Check sheet for the modelled part. Datum: model origin and axes. Units: mm. A direction names the side the tool comes from. Coordinates: 2 decimals unless noted, no trailing zeros. Write each loop counter-clockwise with the first axis right and the second up, starting at its lowest first coordinate (ties: lowest second). Pieces come first, ordered by that corner, then holes. Notation, with made-up numbers: M -3.5,26.25 L 0.5,26.25 A10 ccw 0.5,32.25 Z; hole C 27,-17 d2. An arc over 180 degrees is marked long. Answer as CSV lines item,"result". Start each with the question number.
Q1. Thickness scan on line 1 along Z through (x, y) = (-22, 0.45); line 2 along X through (y, z) = (2.5, -37.5); line 3 along X through (y, z) = (0.3, -44.5). Record the ranges inside material, lowest first. Write a range as from..to.
Q2. Depth check by flat-ended pin: pin 1 Ø1 at (x, z) = (-9, -41.5) entering from +Y. Enter the tip coordinate at first touch or a pass-through.
Q3. Access from +Z, -Z, +X, -X, +Y, -Y to the whole of each face (thin tool, end or side, straight path). Record for faces 4 (the cylindrical face through (-15.01, 0.49, -33.54)), 5 (the flat face through (-43, 11, -31)).
Q4. Mould release check, pull along X, two halves, no side actions. Record for faces 1 (the flat face through (-17.6, 1, -31.9)), 2 (the flat face through (0, 11, -32)), 3 (the flat face through (-22, 11, -63)): pulls with the +X half, pulls with the -X half, needs draft (parallel to the pull), parting line crosses it, or undercut.
Q5. Sectioned sample at D-D, the plane z = -58.5. Record the cut outline in (x, y), then the cut area to 3 significant figures.
Q6. Sectioned sample at A-A, the plane z = -44.5. Record the cut outline in (x, y), then the cut area to 3 significant figures.
Q7. Sectioned sample at B-B, the plane x = -22. Record the cut outline in (y, z), then the cut area to 3 significant figures.
Q8. Sectioned sample at C-C, the plane y = 9.25. Record the cut outline in (x, z), then the cut area to 3 significant figures.
Autodesk Fusion 360 part; units mm, degrees
sketch "Sketch1" plane through (0, 0, 0) normal (0, 1, 0) x (1, 0, 0)
  line L0 (0, 0) -> (-44, 0)
  line L1 (-44, 0) -> (-44, 63)
  line L2 (-44, 63) -> (0, 63)
  line L3 (0, 63) -> (0, 0)
  line L4 (-22, 0) -> (-22, 15)
  line L5 (-44, 0) -> (-22, 0)
  line L6 (-22, 0) -> (-22, 63)
  line L7 (-22, 63) -> (-22, 44.5)
  circle A0 centre (-22, 44.5) radius 13
  line L8 (-44, 63) -> (-22, 63)
  line L9 (-5.2012, 3.5077) -> (-38.7988, 3.5077)
  line L10 (-38.7988, 3.5077) -> (-38.7988, 26.4923)
  line L11 (-38.7988, 26.4923) -> (-5.2012, 26.4923)
  line L12 (-5.2012, 26.4923) -> (-5.2012, 3.5077)
  line L13 (-5.2012, 3.5077) -> (-38.7988, 26.4923) construction
  line L14 (-38.7988, 3.5077) -> (-5.2012, 26.4923) construction
  line L15 (-43, 62) -> (-1, 62)
  line L16 (-1, 62) -> (-1, 1)
  line L17 (-1, 1) -> (-43, 1)
  line L18 (-43, 1) -> (-43, 62)
  dimension "d1" = 44
  dimension "d2" = 63
  dimension "d5" = 15
  dimension "d7" = 18.5
  dimension "d8" = 26
  dimension "d9" = 21
  dimension "d13" = 21.5
  dimension "d14" = 1
extrude "Extrude3" add sketch "Sketch1" along normal blind 22 contours L0 L2 L3 L4 L6 L7 L15 L16 L17 | L0 L1 L2 L4 L5 L6 L7 L8 L15 L17 L18 makes body 1
extrude "Extrude2" add sketch "Sketch1" along normal blind 1 separate body contours L0 L2 L3 L4 L6 L7 L15 L16 L17 | L0 L1 L2 L4 L5 L6 L7 L8 L15 L17 L18 | L4 L6 L7 A0 L9 L10 L11 L15 L17 L18 | L4 L6 L7 A0 L9 L11 L12 L15 L16 L17 makes body 2
combine "Combine1" operation add target body 1 tool bodies 2
extrude "Extrude5" add sketch "Sketch1" along normal blind 21 separate body contours L4 L6 L7 A0 L9 L10 L11 L15 L17 L18 | L4 L6 L7 A0 L9 L11 L12 L15 L16 L17 | L4 L6 L9 L10 L11 | L4 L6 L9 L11 L12 | L6 L7 A0 | L6 L7 A0 makes body 3
move_body "Move1" bodies 3 to x (1, 0, 0) y (0, 1, 0) z (0, 0, 1) at (0, 1, 0)
extrude "Extrude6" add sketch "Sketch1" along normal blind -8 and the other way blind -1 separate body contours L6 L7 A0 | L6 L7 A0 makes body 4
combine "Combine2" operation add target body 4 tool bodies 3
sketch "Sketch3" plane through (0, 0, 0) normal (1, 0, 0) x (0, 0, -1)
  line L0 (44.5, -8) -> (44.5, -95.3333)
  line L1 (44.5, -8) -> (44.5007, 25.9882)
  line L2 (44.5, -8) -> (44.5, -13)
  line L3 (44.5, -8) -> (44.5, -13)
  line L4 (44.5, -8) -> (44.5, -13)
  line L5 (44.5, -5.7455) -> (28.5885, -9.273)
  line L6 (44.5, -5.7455) -> (93.193, -5.7455) construction
  line L7 (44.5, -5.7455) -> (101.0974, -5.7455) construction
  line L8 (44.5, -9.273) -> (25, -9.273)
  line L9 (28.5885, -9.273) -> (28.5885, -28.9115)
  line L10 (28.5885, -28.9115) -> (23.5129, -33.9871)
  line L11 (44.5, -13) -> (73.6492, -13) construction
  line L12 (44.5, -13) -> (28.5885, -28.9115)
  line L13 (28.5885, -28.9115) -> (-8.934, -28.9115)
  line L14 (44.5, -13) -> (28.5885, -13)
  line L15 (44.5, -13) -> (7, -12.9775)
  line L16 (7, -12.9775) -> (30.0264, -12.9775) construction
  line L17 (7, -12.9775) -> (-8.934, -28.9115)
  line L18 (-8.934, -28.9115) -> (-8.934, -33.9115)
  line L19 (6.9775, -13) -> (6.9775, -33.9115)
  line L20 (28.5885, -13) -> (6.9775, -13)
  line L21 (-8.934, -28.9115) -> (-8.934, -33.9115)
  line L22 (-8.934, -33.9115) -> (6.9775, -33.9115)
  line L23 (6.9775, -33.9115) -> (44.5, -42.23)
  line L24 (6.9775, -33.9115) -> (31.1364, -33.9115) construction
  line L25 (-8.934, -33.9115) -> (-89.4653, -51.7648)
  line L26 (-8.934, -33.9115) -> (73.5526, -33.9115) construction
  dimension "d31" = 5
  dimension "d36" = 45
  dimension "d37" = 77.5
  dimension "d38" = 37.5
  dimension "d40" = 12.5
  dimension "d41" = 167.5
sketch "Sketch4" plane through (0, 0, 0) normal (1, 0, 0) x (0, 0, -1)
  line L0 (63, 0) -> (44.5, 0)
  line L1 (44.5, 0) -> (44.5, -81.2522)
  line L2 (31.5, -8) -> (57.5, -8)
  line L3 (44.5, -8) -> (57, -8)
  line L4 (44.5, -6.4048) -> (93.5414, -6.4048) construction
  line L5 (44.5, -8) -> (44.5, -13)
  line L6 (44.5, -8) -> (31.5, -8)
  line L7 (31.5, -8) -> (34.5, -8)
  line L8 (44.5, -6.3277) -> (113.977, -6.3277) construction
  line L9 (44.5, -9.2652) -> (31.25, -9.2652)
  line L10 (31.25, -9.2652) -> (31.25, -24.1181)
  line L11 (44.5, -13) -> (31.25, -24.1181)
  line L12 (44.5, -13) -> (64.8642, -13) construction
  line L13 (44.5, -13) -> (7, -6.3877)
  line L14 (57.3025, -15.2574) -> (44.5, -13)
  line L15 (45.8772, -26.6972) -> (-6.25, -17.5058)
  line L16 (44.5, 0) -> (7, 0)
  line L17 (7, -6.3877) -> (7, -30)
  line L18 (7, -6.3877) -> (-6.25, -17.5058)
  line L19 (7, -6.3877) -> (33.2311, -6.3877) construction
  line L20 (44.5, -6.3277) -> (7, -14.6413)
  line L21 (-6.25, -17.5058) -> (-6.25, -43.4537)
  line L22 (7, -14.6413) -> (7, -36.5614)
  line L23 (7, -6.3877) -> (7, -14.6413)
  dimension "d44" = 5
  dimension "d46" = 3
  dimension "d47" = 167.5
  dimension "d49" = 50
  dimension "d50" = 37.5
  dimension "d51" = 140
hidden bodies 4
Output:
1,line 1,"z = -63..-57.5, -31.5..-26.49, -3.51..0"
1,line 2,"x = -44..-43, -1..0"
1,line 3,"x = -44..-35, -9..0"
2,pin 1,"stops at y = 1"
3,face 4,"+Y, -Y"
3,face 5,"+Y"
4,face 1,"undercut"
4,face 2,"pulls with the +X half"
4,face 3,"needs draft"
5,outline,"M -44,0 L 0,0 L 0,22 L -1,22 L -1,1 L -43,1 L -43,22 L -44,22 Z"
5,area,"86.0 mm^2"
6,outline,"M -44,0 L -35,0 L -35,1 L -43,1 L -43,22 L -44,22 Z; M -9,0 L 0,0 L 0,22 L -1,22 L -1,1 L -9,1 Z"
6,area,"60.0 mm^2"
7,outline,"M 0,-63 L 22,-63 L 22,-62 L 1,-62 L 1,-57.5 L 0,-57.5 Z; M 0,-31.5 L 1,-31.5 L 1,-26.49 L 0,-26.49 Z; M 0,-3.51 L 1,-3.51 L 1,-1 L 22,-1 L 22,0 L 0,0 Z"
7,area,"56.0 mm^2"
8,outline,"M -44,-63 L 0,-63 L 0,0 L -44,0 Z; hole M -43,-62 L -1,-62 L -1,-1 L -43,-1 Z"
8,area,"210 mm^2"
